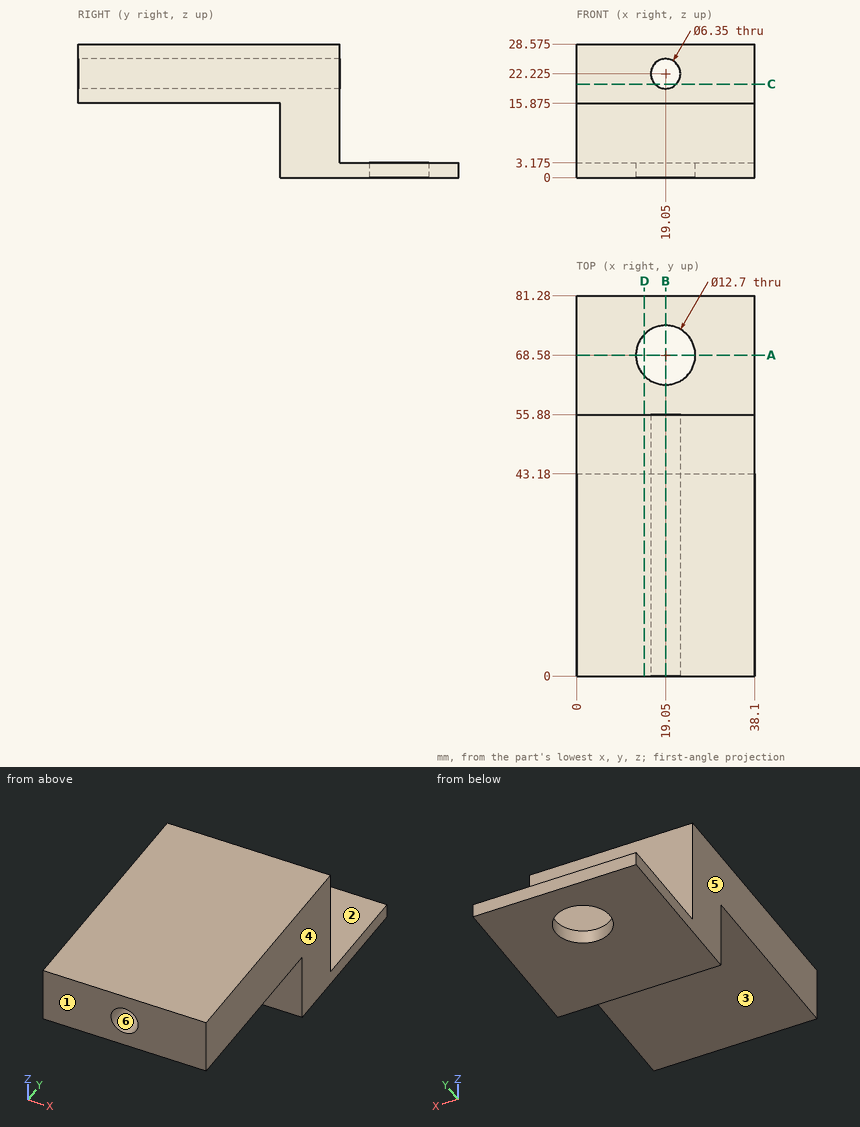
Design review of the part shown in the three views and the two pictorial views. Dimensions are in mm from the part's minimum x, y and z. A direction names the side the tool comes from. Round coordinates to 2 decimals unless told otherwise and drop trailing zeros. Loops run counter-clockwise (first coordinate to the right, second up) from the corner with the lowest first, then second, coordinate; pieces in that order, holes last. Notation, with made-up numbers: (-39.5, 73.5) - (17.5, 73.5) arc R24 cw to (17.5, 89.5) - close; hole circle Ø3 at (40.5, -0.5). An arc over 180 degrees is marked (long way). One line per item, written item: value. Start each with the question number.
Item 1: Take a section at C-C (z = 20). Give the boundary of the cut face in (x, y).
Item 2: Take a section at A-A (y = 68.58). Give the boundary of the cut face in (x, z) (3 decimals).
Item 3: For the marked faces 1, 2 and 3, list the 3-axis set-ups (+Z, -Z, +X, -X, +Y, -Y) from which the entire face can be reached by the end or side of a thin tool; tool diameter is ignored.
Item 4: Clearance check with flat-ended pins moving along their axes: pin 1 Ø4 at (x, z) = (14.5, 10) entering from +Y; pin 2 Ø8 at (x, y) = (16, 10.5) entering from -Z (3 decimals); pin 3 Ø7.5 at (x, y) = (12, 71.5) entering from +Z (3 decimals). State where each tip first meets the part, or that it passes through.
Item 5: The part is to be moulded in two halves that separate along X. For the marked faces 4, 5 and 6, say which applies: +X half, -X half, draft (parallel to the pull), parting line (faces both ways), or undercut.
Item 6: For L1, parallel to Y at x = 19.05, z = 1; L2, parallel to Z at x = 19.05, y = 31.5 (3 decimals); L3, parallel to Z at x = 12, y = 27.5 (3 decimals), list the stretches that pass through material, from the lowest coordinate up.
Item 7: Take a section at B-B (x = 19.05). Give the boundary of the cut face in (y, z) (3 decimals).
Item 8: Take a section at D-D (x = 14.5). Give the boundary of the cut face in (y, z) (3 decimals).
Answer below:
1. outline: (0, 0) - (16.79, 0) - (16.79, 55.88) - (0, 55.88) - close; (21.31, 0) - (38.1, 0) - (38.1, 55.88) - (21.31, 55.88) - close
2. outline: (0, 0) - (12.7, 0) - (12.7, 3.175) - (0, 3.175) - close; (25.4, 0) - (38.1, 0) - (38.1, 3.175) - (25.4, 3.175) - close
3. face 1: +Z, -Z, +X, -X, -Y
3. face 2: +Z, +X, -X, +Y
3. face 3: -Z, +X, -X, -Y
4. pin 1: stops at y = 55.88
4. pin 2: stops at z = 15.875
4. pin 3: stops at z = 3.175
5. face 4: +X half
5. face 5: -X half
5. face 6: undercut
6. L1: y = 43.18 to 62.23, 74.93 to 81.28
6. L2: z = 15.875 to 19.05, 25.4 to 28.575
6. L3: z = 15.875 to 28.575
7. outline: (0, 15.875) - (43.18, 15.875) - (43.18, 0) - (62.23, 0) - (62.23, 3.175) - (55.88, 3.175) - (55.88, 19.05) - (0, 19.05) - close; (0, 25.4) - (55.88, 25.4) - (55.88, 28.575) - (0, 28.575) - close; (74.93, 0) - (81.28, 0) - (81.28, 3.175) - (74.93, 3.175) - close
8. outline: (0, 15.875) - (43.18, 15.875) - (43.18, 0) - (64.151, 0) - (64.151, 3.175) - (55.88, 3.175) - (55.88, 28.575) - (0, 28.575) - close; (73.009, 0) - (81.28, 0) - (81.28, 3.175) - (73.009, 3.175) - close
